```python
from build123d import *

# Parameters (mm, degrees)
BOSS_EXTRUDE3_DEPTH   = 100
BODY_MOVE_COPY2_ANGLE = 90


with BuildPart() as part:
    # Sketch4 → Boss-Extrude3 (new body)
    with BuildSketch(Plane(origin=(0, 0, 0), x_dir=(1, 0, 0), z_dir=(0, 1, 0))):
        with BuildLine():
            Line((-280, 200), (280, 200))
            ThreePointArc((280, 200), (294.142135624, 194.142135624), (300, 180))
            Line((300, 180), (300, -180))
            ThreePointArc((300, -180), (294.142135624, -194.142135624), (280, -200))
            Line((280, -200), (-280, -200))
            ThreePointArc((-280, -200), (-294.142135624, -194.142135624), (-300, -180))
            Line((-300, -180), (-300, 180))
            ThreePointArc((-300, 180), (-294.142135624, 194.142135624), (-280, 200))
        make_face()
    extrude(amount=BOSS_EXTRUDE3_DEPTH)

    # Loft1: read off the stored shape, not the designer's step
    # Loft1: loft between two sections, ruled curve by curve
    loft1_from = [
        Edge.make_bspline([(94.538797531, 700, 81.776621117), (-69.014444703, 700, 270.85421618), (-258.092039765, 700, 107.300973946), (-94.538797531, 700, -81.776621117), (69.014444703, 700, -270.85421618), (258.092039765, 700, -107.300973946), (94.538797531, 700, 81.776621117)], [0, 0, 0, 0, 0.5, 0.5, 0.5, 1, 1, 1, 1], 3, [1, 0.333333333, 0.333333333, 1, 0.333333333, 0.333333333, 1]),
    ]
    loft1_to = [
        Edge.make_bspline([(67.762458695, 100, 133.821706728), (-199.880954762, 100, 269.346624118), (-335.405872151, 100, 1.703210661), (-67.762458695, 100, -133.821706728), (199.880954762, 100, -269.346624118), (335.405872151, 100, -1.703210661), (67.762458695, 100, 133.821706728)], [0, 0, 0, 0, 0.5, 0.5, 0.5, 1, 1, 1, 1], 3, [1, 0.333333333, 0.333333333, 1, 0.333333333, 0.333333333, 1]),
    ]
    loft1 = Solid(Shell([*[Face.make_surface_from_curves(loft1_from[k], loft1_to[k]) for k in range(1)], Face(Wire(loft1_from)), Face(Wire(loft1_to))]))
    add(loft1)


with BuildPart() as part_1:
    # Body-Move/Copy2: moved
    add(part.part.rotate(Axis((0, 0, 0), (1, 0, 0)), BODY_MOVE_COPY2_ANGLE))


solid = part_1.part
```
Design review of the part built by this model. Coordinates are the model's own, in mm. A direction names the side the tool comes from. Coordinates: 2 decimals unless noted, no trailing zeros. Order: outer loops, then holes, each group sorted by start corner. A loop starts at its lowest first (then second) coordinate and runs counter-clockwise, first axis right, second up. Notation, with made-up numbers: M -33,67 L -10,67 A11 cw -10,74 Z; hole C 6.25,-9.5 d4. An arc over 180 degrees is marked long. Answer as a JSON object with one key per item and string values. Group by question number.
1) Tool access review of faces 1 (the flat face through (-4, 200, 49)), 2 (the flat face through (-144, 64, 100)): name each direction out of +Z, -Z, +X, -X, +Y, -Y from which nothing blocks a thin tool from reaching the whole face with its end or side.
2) For pin 1 (6 mm diameter, centred on y = -20.5, z = 294, fed in from -X); pin 2 (12 mm diameter, centred on x = -61.5, z = 207, fed in from -Y); pin 3 (5 mm diameter, centred on x = -154, y = 17, fed in from +Z), all flat-tipped, find the tip position at first contact; note any pin that passes through.
3) Add section A-A, the plane y = 161. Write out the cut boundary in (x, z).
4) Add section B-B, the plane x = -180.5. Write out the cut boundary in (y, z).
5) Wall thickness on L1, parallel to Z at x = 159.5, y = -148; L2, parallel to X at y = 13, z = 344; L3, parallel to Y at x = -83, z = 356: over which ranges is each line inside the solid? List them lowest first.
Computed values:
{
 "1": {"face 1": "+Z, -Z, +X, -X, +Y", "face 2": "+Z"},
 "2": {"pin 1": "stops at x = -138.67", "pin 2": "stops at y = -133.03", "pin 3": "stops at z = 100"},
 "3": {"outline": "M -300,0 L 300,0 L 300,100 L -300,100 Z"},
 "4": {"outline": "M -200,0 L 200,0 L 200,100 L -200,100 Z"},
 "5": {"L1": "z = 0 to 100", "L2": "x = -136.78 to 136.78", "L3": "y = -108.81 to 108.81"}
}
